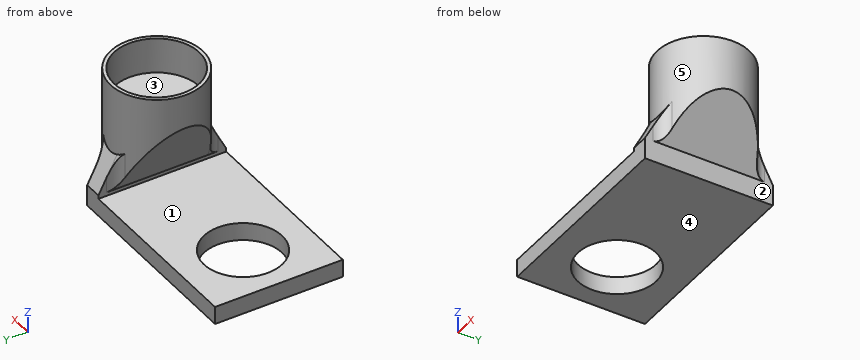
```python
from build123d import *

# Parameters (mm, degrees)
SZKIC1_W                     = 18
SZKIC1_H                     = 18
DODANIE_WYCI_GNI_CIE1_DEPTH  = 2.5
SZKIC3_R                     = 6.5
SZKIC3_R_2                   = 6
DODANIE_WYCI_GNI_CIE2_DEPTH  = 5
SZKIC5_R                     = 6.5
DODANIE_WYCI_GNI_CIE3_DEPTH  = 9.5
SZKIC6_W                     = 2.5
SZKIC6_H                     = 18
DODANIE_WYCI_GNI_CIE4_DEPTH  = 3
WYTNIJ_WYCI_GNI_CIE3_DEPTH   = 20
DODANIE_WYCI_GNI_CIE11_DEPTH = 2.5
ZAOKR_GLENIE3_R              = 2
ZAOKR_GLENIE4_R              = 2
ZAOKR_GLENIE5_R              = 2
ZAOKR_GLENIE6_R              = 2
SZKIC21_W                    = 2.5
SZKIC21_H                    = 18
DODANIE_WYCI_GNI_CIE12_DEPTH = 8
SZKIC23_R                    = 5.5
WYTNIJ_WYCI_GNI_CIE4_DEPTH   = 2.5


with BuildPart() as part:
    # Szkic1 → Dodanie-wyci_gni_cie1 (new body)
    with BuildSketch(Plane.XY):
        with Locations((9, -9)):
            Rectangle(SZKIC1_W, SZKIC1_H)
    extrude(amount=DODANIE_WYCI_GNI_CIE1_DEPTH)

    # Szkic6 → Dodanie-wyci_gni_cie4 (add)
    with BuildSketch(Plane(origin=(0, 0, 0), x_dir=(-1, 0, 0), z_dir=(0, 0, -1))):
        with Locations((-19.25, -9)):
            Rectangle(SZKIC6_W, SZKIC6_H)
    extrude(amount=-DODANIE_WYCI_GNI_CIE4_DEPTH)



with BuildPart() as body_2:
    # Szkic3 → Dodanie-wyci_gni_cie2 (new body)
    with BuildSketch(Plane.XY.offset(12.5)):
        with Locations((19.25, -9)):
            Circle(SZKIC3_R)
        with Locations((19.25, -9)):
            Circle(SZKIC3_R_2, mode=Mode.SUBTRACT)
    extrude(amount=DODANIE_WYCI_GNI_CIE2_DEPTH)

    # Szkic5 → Dodanie-wyci_gni_cie3 (add)
    with BuildSketch(Plane.XY.offset(12.5)):
        with Locations((19.25, -9)):
            Circle(SZKIC5_R)
    extrude(amount=-DODANIE_WYCI_GNI_CIE3_DEPTH)

    # Szkic17 → Wytnij-wyci_gni_cie3 (cut)
    with BuildSketch(Plane(origin=(0, 0, 0), x_dir=(1, 0, 0), z_dir=(0, 1, 0))):
        Polygon((20.5, -3), (25.75, -10.25), (25.75, -3), align=None)
        Polygon((18, -3), (12.696843968, -12.75), (12.75, -3), align=None)
    extrude(amount=-WYTNIJ_WYCI_GNI_CIE3_DEPTH, mode=Mode.SUBTRACT)


with BuildPart() as part_1:
    add(part.part)

    add(body_2.part)  # Dodanie-wyci_gni_cie11 merges body 2
    # Szkic19 → Dodanie-wyci_gni_cie11 (add)
    with BuildSketch(Plane(origin=(20.5, 0, 0), x_dir=(0, 0, -1), z_dir=(1, 0, 0))):
        Polygon((-3, -18), (-3, -15.378675411), (-8, -15.378675411), align=None)
        Polygon((-3, 0), (-3, -2.621324589), (-8, -2.621324589), align=None)
    extrude(amount=-DODANIE_WYCI_GNI_CIE11_DEPTH)

    # Zaokr_glenie3
    zaokr_glenie3_edges = [part_1.edges().sort_by_distance(p)[0] for p in [
        (20.5, -15.378675411, 5.5),
    ]]
    fillet(zaokr_glenie3_edges, radius=ZAOKR_GLENIE3_R)

    # Zaokr_glenie4
    zaokr_glenie4_edges = [part_1.edges().sort_by_distance(p)[0] for p in [
        (20.5, -2.621324589, 5.5),
    ]]
    fillet(zaokr_glenie4_edges, radius=ZAOKR_GLENIE4_R)

    # Zaokr_glenie5
    # the kernel refuses this fillet: 2 mm, written as the material it adds along each edge
    with BuildSketch(Plane(origin=(18, -15.378675411, -0.688659063), x_dir=(0, -1, 0), z_dir=(0, 0, 1))) as zaokr_glenie5_piece_1_section:
        with BuildLine():
            CenterArc((1.475463625, -2), ZAOKR_GLENIE5_R, 90, 67.520494391)
            ThreePointArc((-0.372569089, -1.235294118), (-0.155557822, -0.626914348), (0, 0))
            Line((0, 0), (1.475463625, 0))
        make_face()
    zaokr_glenie5_piece_1 = extrude(amount=12.377318126, mode=Mode.PRIVATE)
    zaokr_glenie5_piece_1 = split(zaokr_glenie5_piece_1, bisect_by=Plane(origin=(16.879667194, -15.616046578, 5.059763053), z_dir=(0.878464068971863, 0, 0.47780841299143956)), keep=Keep.TOP, mode=Mode.PRIVATE)
    zaokr_glenie5_piece_1 = split(zaokr_glenie5_piece_1, bisect_by=Plane(origin=(17.729689725, -16.448851128, 5.958711939), z_dir=(0, 0.8856656985010092, -0.46432345460758234)), keep=Keep.TOP, mode=Mode.PRIVATE)
    add(zaokr_glenie5_piece_1)

    # Zaokr_glenie6
    # the kernel refuses this fillet: 2 mm, written as the material it adds along each edge
    with BuildSketch(Plane(origin=(18, -2.621324589, -0.688659063), x_dir=(0, 1, 0), z_dir=(0, 0, 1))) as zaokr_glenie6_piece_1_section:
        with BuildLine():
            CenterArc((1.475463625, 2), ZAOKR_GLENIE6_R, 202.479505609, 67.520494391)
            ThreePointArc((-0.372569089, 1.235294118), (-0.155557822, 0.626914348), (0, 0))
            Line((0, 0), (1.475463625, 0))
        make_face()
    zaokr_glenie6_piece_1 = extrude(amount=12.377318126, mode=Mode.PRIVATE)
    zaokr_glenie6_piece_1 = split(zaokr_glenie6_piece_1, bisect_by=Plane(origin=(17.729689725, -1.551148872, 5.958711939), z_dir=(0, -0.8856656985010092, -0.4643234546075823)), keep=Keep.TOP, mode=Mode.PRIVATE)
    zaokr_glenie6_piece_1 = split(zaokr_glenie6_piece_1, bisect_by=Plane(origin=(16.879667194, -2.383953422, 5.059763053), z_dir=(0.8784640689720787, 0, 0.4778084129910428)), keep=Keep.TOP, mode=Mode.PRIVATE)
    add(zaokr_glenie6_piece_1)

    # Szkic21 → Dodanie-wyci_gni_cie12 (add)
    with BuildSketch(Plane.ZY):
        with Locations((1.25, -9)):
            Rectangle(SZKIC21_W, SZKIC21_H)
    extrude(amount=DODANIE_WYCI_GNI_CIE12_DEPTH)

    # Szkic23 → Wytnij-wyci_gni_cie4 (cut)
    with BuildSketch(Plane.XY.offset(2.5)):
        with Locations((0, -9)):
            Circle(SZKIC23_R)
    extrude(amount=-WYTNIJ_WYCI_GNI_CIE4_DEPTH, mode=Mode.SUBTRACT)


solid = part_1.part
```
CAD build for the part. Positions are in the model's coordinates, mm. Face numbers are marked on the shaded views. A direction names the side the tool comes from. Round coordinates to 2 decimals unless told otherwise and drop trailing zeros. Order: outer loops, then holes, each group sorted by start corner. A loop starts at its lowest first (then second) coordinate and runs counter-clockwise, first axis right, second up.
Q1. Slice it at D-D (y = -6). Write the cut outline in (x, z), and give its area (3 significant figures).
Q2. Wall check: L1, parallel to Y at x = 0, z = 1.6; L2, parallel to Y at x = 19.25, z = 14.15; L3, parallel to Z at x = 2, y = -1. Give the ranges that are in metal, low to high.
Q3. Slice it at B-B (x = 0). Write the cut outline in (y, z).
Q4. Slice it at A-A (y = -9). Write the cut outline in (x, z), and give its area (3 significant figures).
Q5. Slice it at C-C (z = 7.5). Write the cut outline in (x, y), and give its area (3 significant figures).
Q6. Drop flat-ended pins along their axis: pin 1 (6 mm diameter, centred on y = -5, z = 12.5, fed in from +X); pin 2 (6 mm diameter, centred on y = -7, z = 11.5, fed in from -X); pin 3 (2 mm diameter, centred on y = -11, z = 7.5, fed in from -X); pin 4 (5.5 mm diameter, centred on x = 1.5, y = -10.5, fed in from +Z). Give the stop position or say it passes through.
Q7. Two-plate mould, pull along Z, no slides. Class the marked faces 1, 2 and 3: pulls with the +Z half, pulls with the -Z half, needs draft (parallel to the pull), parting line crosses it, or undercut.
Q8. Which spindle directions (+Z, -Z, +X, -X, +Y, -Y) get a long thin tool onto all of the face, cutting with end or side? Do the marked faces 4 and 5. Say none if no direction does.
Results below:
1. outline: (-8, 0) - (-4.61, 0) - (-4.61, 2.5) - (-8, 2.5) - close; (4.61, 0) - (20.5, 0) - (20.5, 3) - (25.02, 9.24) - (25.02, 17.5) - (24.45, 17.5) - (24.45, 12.5) - (14.05, 12.5) - (14.05, 17.5) - (13.48, 17.5) - (13.48, 11.3) - (18, 3) - (18, 2.5) - (4.61, 2.5) - close
1. area: 132 mm2
2. L1: y = -18 to -14.5, -3.5 to 0
2. L2: y = -15.5 to -15, -3 to -2.5
2. L3: z = 0 to 2.5
3. outline: (-18, 0) - (-14.5, 0) - (-14.5, 2.5) - (-18, 2.5) - close; (-3.5, 0) - (0, 0) - (0, 2.5) - (-3.5, 2.5) - close
4. outline: (-8, 0) - (-5.5, 0) - (-5.5, 2.5) - (-8, 2.5) - close; (5.5, 0) - (20.5, 0) - (20.5, 3) - (25.75, 10.25) - (25.75, 17.5) - (25.25, 17.5) - (25.25, 12.5) - (13.25, 12.5) - (13.25, 17.5) - (12.75, 17.5) - (12.75, 12.65) - (18, 3) - (18, 2.5) - (5.5, 2.5) - close
4. area: 129 mm2
5. outline: (15.55, -14.35) arc R6.5 ccw to (16.76, -15.01) arc R2 cw to (17.59, -15.64) - (20.91, -15.64) arc R2 cw to (21.74, -15.01) arc R6.5 ccw to (23.76, -13.68) - (23.76, -4.32) arc R6.5 ccw to (21.74, -2.99) arc R2 cw to (20.91, -2.36) - (17.59, -2.36) arc R2 cw to (16.76, -2.99) arc R6.5 ccw to (15.55, -3.65) - close
5. area: 101 mm2
6. pin 1: stops at x = 25.67
6. pin 2: stops at x = 12.75
6. pin 3: stops at x = 15.01
6. pin 4: passes through
7. face 1: undercut
7. face 2: needs draft
7. face 3: pulls with the +Z half
8. face 4: -Z, +X, -X, +Y, -Y
8. face 5: +Z
